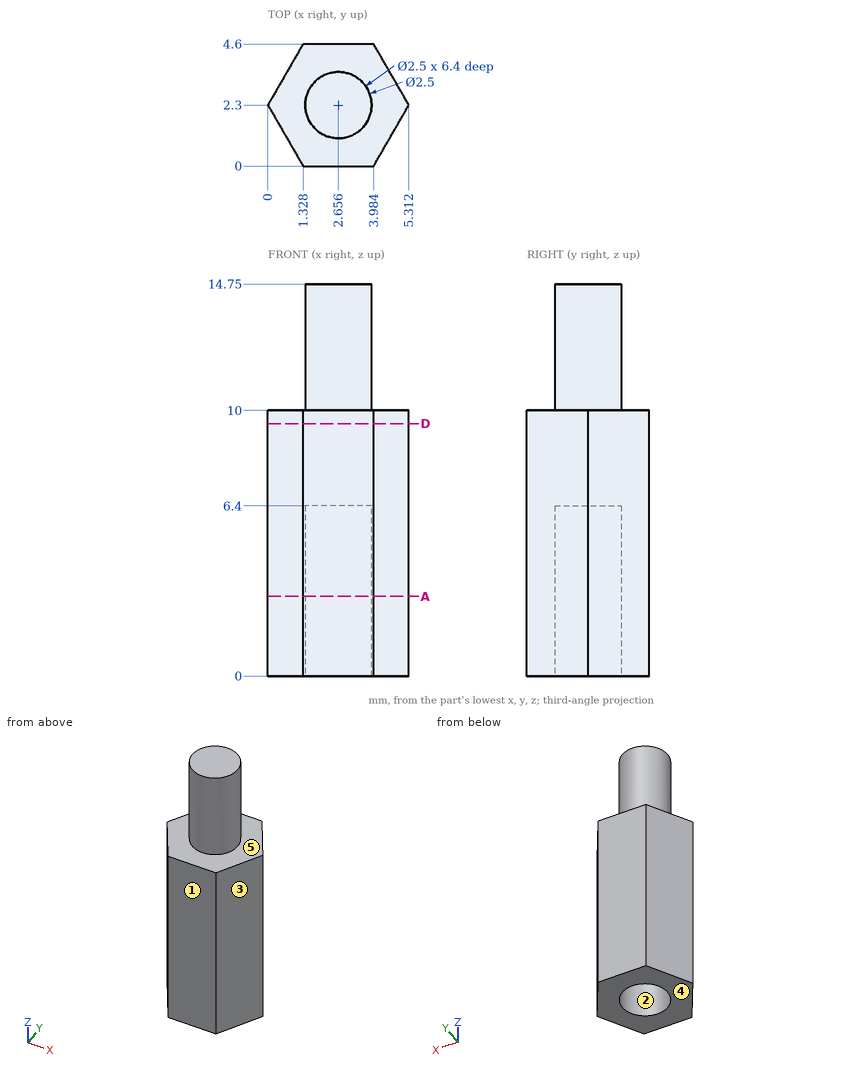
Print and shaded views of the part. All mm, measured from the part's lowest x, y and z. A direction names the side the tool comes from. Coordinates: 2 decimals unless noted, no trailing zeros. Order: outer loops, then holes, each group sorted by start corner. A loop starts at its lowest first (then second) coordinate and runs counter-clockwise, first axis right, second up. Notation, with made-up numbers: (41, 69) - (95, 69) arc R21 cw to (95, 98) - close; hole circle Ø3 at (82.25, 89). An arc over 180 degrees is marked (long way). Return JSON: item names as keys, results as strings. Group by question number.
Item 1: Which spindle directions (+Z, -Z, +X, -X, +Y, -Y) get a long thin tool onto all of the face, cutting with end or side? Do the marked faces 4 and 5. Say none if no direction does.
Item 2: Cut at D-D (z = 9.5). List the corners of the cut face in (x, y).
Item 3: Pin check, flat tips, straight feed: pin 1 (1 mm diameter, centred on x = 2.5, y = 2.5, fed in from -Z); pin 2 (1.5 mm diameter, centred on x = 1, y = 4, fed in from -Z); pin 3 (1 mm diameter, centred on x = 4.5, y = 1, fed in from +Z); pin 4 (1.5 mm diameter, centred on y = 1.5, z = 12, fed in from +X) (1 decimal). Stop position of each tip, or through.
Item 4: Pull direction X, two halves, no side cores. Call the marked faces 1, 2 and 3: pulls with the +X half, pulls with the -X half, needs draft (parallel to the pull), parting line crosses it, or undercut.
Item 5: Drill centre lines: probe 1 along Z at (x, y) = (0.75, 2.65); probe 2 along X at (y, z) = (1.8, 2.5); probe 3 along Z at (x, y) = (1.65, 1.85). Where is each one in solid material? Low to high. Write a range as from..to.
Item 6: Cut at A-A (z = 3). List the corners of the cut face in (x, y).
Check values:
{
 "1": {"face 4": "-Z, +X, -X, +Y, -Y", "face 5": "+Z"},
 "2": {"outline": "(0, 2.3) - (1.33, 0) - (3.98, 0) - (5.31, 2.3) - (3.98, 4.6) - (1.33, 4.6) - close"},
 "3": {"pin 1": "stops at z = 6.4", "pin 2": "stops at z = 0", "pin 3": "stops at z = 10", "pin 4": "stops at x = 3.9"},
 "4": {"face 1": "needs draft", "face 2": "undercut", "face 3": "pulls with the +X half"},
 "5": {"probe 1": "z = 0..10", "probe 2": "x = 0.29..1.51, 3.8..5.02", "probe 3": "z = 6.4..14.75"},
 "6": {"outline": "(0, 2.3) - (1.33, 0) - (3.98, 0) - (5.31, 2.3) - (3.98, 4.6) - (1.33, 4.6) - close; hole circle Ø2.5 at (2.66, 2.3)"}
}
